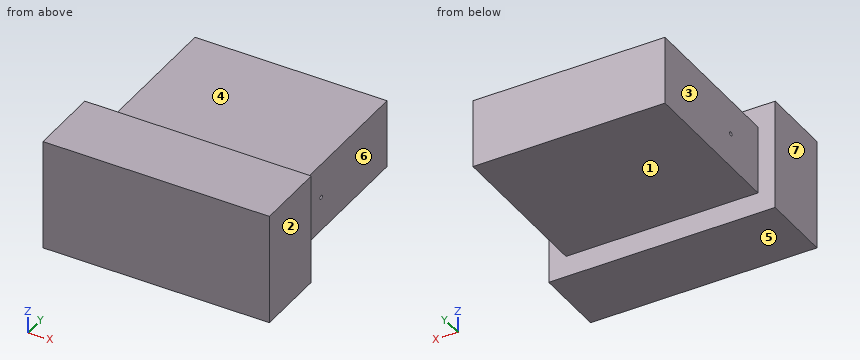
```python
from build123d import *

# Parameters (mm, degrees)
F0_W      = 145
F0_H      = 52
F1_DEPTH  = 120
F0_W_2    = 171
F0_H_2    = 84
F1_FACE_W = 145
F1_FACE_H = 52
F2_DEPTH  = 54
F5_D      = 3


with BuildPart() as f1:
    # F0 (on Front) → F1 (new body)
    with BuildSketch(Plane.XZ):
        with Locations((17.016632, 19.899432)):
            Rectangle(F0_W, F0_H)
    extrude(amount=-F1_DEPTH)

    # F0 (on Front) + F1_face (on face) → F2 (join)
    with BuildSketch(Plane.XZ):
        with Locations((17.016632, 19.899432)):
            Rectangle(F0_W_2, F0_H_2)
        with Locations((17.016632, 19.899432)):
            Rectangle(F0_W, F0_H, mode=Mode.SUBTRACT)
    with BuildSketch(Plane(origin=(17.016632, 0, 19.899432), x_dir=(1, 0, 0), z_dir=(0, -1, 0))):
        Rectangle(F1_FACE_W, F1_FACE_H)
    extrude(amount=F2_DEPTH)

    # F5 (through all)
    with Locations(Plane.YZ.offset(90)):
        with Locations((35, 19.899432)):
            Hole(F5_D / 2)


solid = f1.part
```
Input: part model. Units: mm. Frame: model coordinates. Face numbers are marked on the shaded views. A direction names the side the tool comes from. Round coordinates to 2 decimals unless told otherwise and drop trailing zeros. Loops run counter-clockwise (first coordinate to the right, second up) from the corner with the lowest first, then second, coordinate; pieces in that order, holes last. Notation, with made-up numbers: (54.5, -11) - (92.5, -11) arc R14 ccw to (92.5, 6) - close; hole circle Ø8 at (4.25, 23). An arc over 180 degrees is marked (long way). One line per item, written item: value. Start each with the question number.
(1) Section A-A, the plane x = -40. Return loops of the section in (y, z).
(2) Section D-D, the plane z = -12. Return loops of the section in (x, y), plus the area to 3 significant figures.
(3) Ray query, line 1 (Z direction, x = -11.5, y = 35); line 2 (X direction, y = 62, z = 34); line 3 (Y direction, x = 55, z = 49). Return the intervals inside material, ascending. Write a range as [from, to].
(4) Access query for the marked faces 1, 2, 3 and 4. Directions: +Z, -Z, +X, -X, +Y, -Y. A direction counts if a zero-diameter tool reaches every point of the face in a straight line with its end or side. Return the directions, or none.
(5) Draft query along X for the marked faces 5, 6 and 7. Return one class per face: +X half, -X half, draft (parallel to the pull), parting line (faces both ways), or undercut.
(6) Section C-C, the plane y = 42. Return loops of the section in (x, z), plus the area to 3 significant figures.
(7) Contact query for flat-ended pins moving along their axis: P1, Ø5, axis at x = -6, y = 8.5, coming from the +Z side; P2, Ø6, axis at y = 2, z = 12, coming from the -X side; P3, Ø2.5, axis at y = 35, z = 19.9, coming from the +X side. Output: stop coordinate, or through.
(8) Section B-B, the plane z = 39. Return loops of the section in (x, y).
Results below:
1. outline: (-54, -22.1) - (0, -22.1) - (0, -6.1) - (120, -6.1) - (120, 45.9) - (0, 45.9) - (0, 61.9) - (-54, 61.9) - close; hole circle Ø3 at (35, 19.9)
2. outline: (-68.48, -54) - (102.52, -54) - (102.52, 0) - (-68.48, 0) - close
2. area: 9,230 mm^2
3. line 1: [-6.1, 18.4], [21.4, 45.9]
3. line 2: [-55.48, 89.52]
3. line 3: [-54, 0]
4. face 1: -Z, +X, -X, +Y
4. face 2: +Z, -Z, +X, +Y, -Y
4. face 3: +Z, -Z, -X, +Y
4. face 4: +Z, +X, -X, +Y
5. face 5: draft
5. face 6: +X half
5. face 7: -X half
6. outline: (-55.48, -6.1) - (89.52, -6.1) - (89.52, 45.9) - (-55.48, 45.9) - close
6. area: 7,540 mm^2
7. P1: z = 45.9
7. P2: x = -68.48
7. P3: through
8. outline: (-68.48, -54) - (102.52, -54) - (102.52, 0) - (89.52, 0) - (89.52, 120) - (-55.48, 120) - (-55.48, 0) - (-68.48, 0) - close
